Geometry: final body of the model. Coordinates: model frame, mm. Coordinates: 2 decimals unless noted, no trailing zeros. Order: outer loops, then holes, each group sorted by start corner. A loop starts at its lowest first (then second) coordinate and runs counter-clockwise, first axis right, second up. Notation, with made-up numbers: (43, 51.25) -> (48, 51.25) arc R25 cw to (48, 90.25) -> close; hole circle Ø1 at (14, 69.5). An arc over 180 degrees is marked (long way). Use CSV: the item, a comma, the result in double quotes. Start each with the question number.
Autodesk Inventor part; units mm, degrees
ref_plane "YZ Plane" through (0, 0, 0) normal (1, 0, 0) x (0, 1, 0)
ref_plane "XZ Plane" through (0, 0, 0) normal (0, 1, 0) x (-1, 0, 0)
ref_plane "XY Plane" through (0, 0, 0) normal (0, 0, 1) x (1, 0, 0)
sketch "Эскиз1" plane through (0, 0, 0) normal (0, 1, 0) x (-1, 0, 0)
  line L0 (125, 125) -> (-125, 125)
  line L1 (-125, 125) -> (-125, -125)
  line L2 (-125, -125) -> (125, -125)
  line L3 (125, -125) -> (125, 125)
  line L4 (125, 125) -> (-125, -125) construction
  line L5 (-125, 125) -> (125, -125) construction
  point P0 (0, 0)
  dimension "d0" = 250
  dimension "d1" = 250
extrude "Выдавливание1" add sketch "Эскиз1" along normal mid plane 4
sketch "Эскиз2" plane through (0, -2, 0) normal (0, -1, 0) x (1, 0, 0)
  line L0 (104.5, -110) -> (104.5, -100)
  line L1 (104.5, -100) -> (94.5, -100)
  line L2 (94.5, -100) -> (94.5, -110)
  line L3 (94.5, -110) -> (104.5, -110)
  circle A0 centre (99.5, -85) radius 2
  line L4 (104.5, -70) -> (104.5, -60)
  line L5 (104.5, -60) -> (94.5, -60)
  line L6 (94.5, -60) -> (94.5, -70)
  line L7 (94.5, -70) -> (104.5, -70)
  circle A1 centre (99.5, -45) radius 2
  line L8 (104.5, -30) -> (104.5, -20)
  line L9 (104.5, -20) -> (94.5, -20)
  line L10 (94.5, -20) -> (94.5, -30)
  line L11 (94.5, -30) -> (104.5, -30)
  circle A2 centre (99.5, -5) radius 2
  line L12 (104.5, 10) -> (104.5, 20)
  line L13 (104.5, 20) -> (94.5, 20)
  line L14 (94.5, 20) -> (94.5, 10)
  line L15 (94.5, 10) -> (104.5, 10)
  circle A3 centre (99.5, 35) radius 2
  line L16 (94.5, 55) -> (94.5, 50)
  line L17 (94.5, 50) -> (104.5, 50)
  line L18 (104.5, 50) -> (104.5, 55)
  line L19 (104.5, 55) -> (104.5, 60)
  line L20 (104.5, 60) -> (94.5, 60)
  line L21 (94.5, 60) -> (94.5, 55)
  line L22 (104.5, 90) -> (104.5, 100)
  line L23 (104.5, 100) -> (94.5, 100)
  line L24 (94.5, 100) -> (94.5, 90)
  line L25 (94.5, 90) -> (104.5, 90)
  line L26 (-104.5, 90) -> (-104.5, 100)
  line L27 (-94.5, 90) -> (-104.5, 90)
  line L28 (-94.5, 100) -> (-94.5, 90)
  line L29 (-104.5, 100) -> (-94.5, 100)
  line L30 (-104.5, 50) -> (-104.5, 55)
  line L31 (-94.5, 50) -> (-104.5, 50)
  line L32 (-94.5, 55) -> (-94.5, 50)
  line L33 (-94.5, 60) -> (-94.5, 55)
  line L34 (-104.5, 60) -> (-94.5, 60)
  line L35 (-104.5, 55) -> (-104.5, 60)
  line L36 (-104.5, 10) -> (-104.5, 20)
  line L37 (-94.5, 10) -> (-104.5, 10)
  line L38 (-94.5, 20) -> (-94.5, 10)
  line L39 (-104.5, 20) -> (-94.5, 20)
  line L40 (-104.5, -30) -> (-104.5, -20)
  line L41 (-94.5, -30) -> (-104.5, -30)
  line L42 (-94.5, -20) -> (-94.5, -30)
  line L43 (-104.5, -20) -> (-94.5, -20)
  line L44 (-104.5, -70) -> (-104.5, -60)
  line L45 (-94.5, -70) -> (-104.5, -70)
  line L46 (-94.5, -60) -> (-94.5, -70)
  line L47 (-104.5, -60) -> (-94.5, -60)
  line L48 (-104.5, -110) -> (-104.5, -100)
  line L49 (-94.5, -110) -> (-104.5, -110)
  line L50 (-94.5, -100) -> (-94.5, -110)
  line L51 (-104.5, -100) -> (-94.5, -100)
  circle A4 centre (-99.5, -85) radius 2
  circle A5 centre (-99.5, -45) radius 2
  circle A6 centre (-99.5, -5) radius 2
  circle A7 centre (-99.5, 35) radius 2
  circle A8 centre (-99.5, 75) radius 2
  circle A9 centre (99.5, 75) radius 2
extrude "Выдавливание2" cut sketch "Эскиз2" against normal up to surface (4 mm away)
sketch "Эскиз3" plane through (0, -2, 0) normal (0, -1, 0) x (1, 0, 0)
  circle A0 centre (75, -95) radius 3.15
  line L0 (125, -125) -> (125, 125)
  line L1 (-125, -125) -> (125, -125)
  line L2 (0, -76.118) -> (0, 76.118) construction
  line L3 (24.9561, 0) -> (-24.9561, 0) construction
  circle A1 centre (-75, -95) radius 3.15
  line L4 (-24.9561, 0) -> (24.9561, 0) construction
  circle A2 centre (75, 95) radius 3.15
  circle A3 centre (-75, 95) radius 3.15
  point P0 (0, 0)
  point P1 (0, 0)
  dimension "d10" = 6.3
  dimension "d14" = 50
  dimension "d15" = 30
extrude "Выдавливание3" cut sketch "Эскиз3" against normal up to surface (4 mm away)
sketch "Эскиз4" plane through (0, -2, 0) normal (0, -1, 0) x (1, 0, 0)
  circle A0 centre (-8, 44.7403) radius 1.85
  circle A1 centre (-8, 30.7403) radius 1.85
  circle A2 centre (0, 37.7403) radius 5
  circle A3 centre (8, 44.7403) radius 1.85
  circle A4 centre (8, 30.7403) radius 1.85
  point P0 (0, 0)
extrude "Выдавливание4" cut sketch "Эскиз4" against normal up to surface (4 mm away)
properties part number "Основание подъёмника"
(1) Section C-C (y = -0.3). State how many separate pieces and enclosed holes the cut face has, then the cut area to 3 significant figures.
(2) Section B-B (x = 75). Return loops of the section in (y, z), then the cut area to 3 significant figures.
(3) Section A-A (z = -65). Return loops of the section in (x, y).
(4) Line query: line 1 (X direction, y = -1.45, z = -106.5); line 2 (Z direction, x = -75, y = -0.4); line 3 (Z direction, x = -6.5, y = -0.5). Output: solid intervals per line, ascending. Write a range as from..to.
(5) Mould query, pull axis Z, two halves, no side actions, for faces 1 (the face through (2, -2, 2)), 2 (the face through (72.68, -0.03, -92.87)). Classes: pulls with the +Z half, pulls with the -Z half, needs draft (parallel to the pull), parting line crosses it, or undercut.
Check sheet entries:
1,separate pieces,"1"
1,enclosed holes,"31"
1,area,"60,900 mm^2"
2,outline,"(-2, -125) -> (2, -125) -> (2, -98.15) -> (-2, -98.15) -> close; (-2, -91.85) -> (2, -91.85) -> (2, 91.85) -> (-2, 91.85) -> close; (-2, 98.15) -> (2, 98.15) -> (2, 125) -> (-2, 125) -> close"
2,area,"950 mm^2"
3,outline,"(-125, -2) -> (-104.5, -2) -> (-104.5, 2) -> (-125, 2) -> close; (-94.5, -2) -> (94.5, -2) -> (94.5, 2) -> (-94.5, 2) -> close; (104.5, -2) -> (125, -2) -> (125, 2) -> (104.5, 2) -> close"
4,line 1,"x = -125..-104.5, -94.5..94.5, 104.5..125"
4,line 2,"z = -125..-98.15, -91.85..91.85, 98.15..125"
4,line 3,"z = -125..29.66, 31.82..43.66, 45.82..125"
5,face 1,"needs draft"
5,face 2,"undercut"
